Autodesk Inventor part; units mm, degrees
ref_plane "Start Plane" through (0, 0, 20) normal (0, 0, 1) x (1, 0, 0)
ref_plane "End Plane" through (0, 0, 1180) normal (0, 0, 1) x (1, 0, 0)
ref_plane "Work Plane4" through (-800, -15.5, 20) normal (0, 0, -1) x (-1, 0, 0)
ref_plane "Start Plane" through (0, 0, 20) normal (0, 0, 1) x (1, 0, 0)
ref_plane "End Plane" through (0, 0, 1180) normal (0, 0, 1) x (1, 0, 0)
sketch "Sketch" plane through (0, 0, 0) normal (0, 0, 1) x (1, 0, 0)
  line L0 (-20, -15.5) -> (-20, 15.5)
  line L1 (-15.5, 20) -> (15.5, 20)
  line L2 (20, 15.5) -> (20, -15.5)
  line L3 (15.5, -20) -> (-15.5, -20)
  arc A0 (-20, -15.5) -> (-15.5, -20) centre (-15.5, -15.5) ccw
  arc A1 (-15.5, 20) -> (-20, 15.5) centre (-15.5, 15.5) ccw
  arc A2 (20, 15.5) -> (15.5, 20) centre (15.5, 15.5) ccw
  arc A3 (15.5, -20) -> (20, -15.5) centre (15.5, -15.5) ccw
  arc A4 (-15.5, 17) -> (-17, 15.5) centre (-15.5, 15.5) ccw
  line L4 (-15.5, 17) -> (15.5, 17)
  arc A5 (17, 15.5) -> (15.5, 17) centre (15.5, 15.5) ccw
  line L5 (17, 15.5) -> (17, -15.5)
  arc A6 (15.5, -17) -> (17, -15.5) centre (15.5, -15.5) ccw
  line L6 (15.5, -17) -> (-15.5, -17)
  arc A7 (-17, -15.5) -> (-15.5, -17) centre (-15.5, -15.5) ccw
  line L7 (-17, -15.5) -> (-17, 15.5)
  line L8 (0, 29.3048) -> (0, -29.3048) construction
  line L9 (-29.3048, 0) -> (29.3048, 0) construction
  dimension "d7" = 4.5
  dimension "d10" = 40
  dimension "d11" = 40
  dimension "d12" = 3
  dimension "d15" = 20
  dimension "d16" = 20
extrude "Body" add sketch "Sketch" along normal up to surface (1160 mm away) from surface at 20
sketch "Sketch3" plane through (0, 0, 0) normal (0, 0, 1) x (1, 0, 0)
  line L0 (0, 0) -> (10, 0)
ref_plane "Work Plane3" through (0, 0, 0) normal (0, -1, 0) x (1, 0, 0)
ref_plane "Work Plane4" through (-800, -15.5, 20) normal (0, 0, -1) x (-1, 0, 0)
split "Split1" plane through (-800, -15.5, 20) removes the side toward (0, 0, -1)
ref_plane "Work Plane5" through (-500, -984.5, 1180) normal (0, 0, 1) x (1, 0, 0)
split "Split2" plane through (-500, -984.5, 1180) removes the side toward (0, 0, 1)
sketch "Sketch4" plane through (0, 0, 0) normal (0, -1, 0) x (1, 0, 0)
  line L0 (-2, 20) -> (12, 20)
  line L1 (-2, 1180) -> (12, 1180)
  dimension "d18" = 1160
equation "\"d7\" = G_IR"
equation "\"d10\" = G_H"
equation "\"d11\" = G_W"
equation "\"d12\" = G_T"
equation "\"d15\" = 0.5 * d10"
equation "\"d16\" = 0.5 * d11"
equation "\"d3\" = G_L"
equation "\"G_W\" = 40"
equation "\"G_H\" = 40"
equation "\"G_T\" = 3"
equation "\"G_IR\" = 4.5"
equation "\"G_L\" = d18"
properties part number "ISO 12633-2 - 40x40x3 - 1160" material "Steel, Mild"
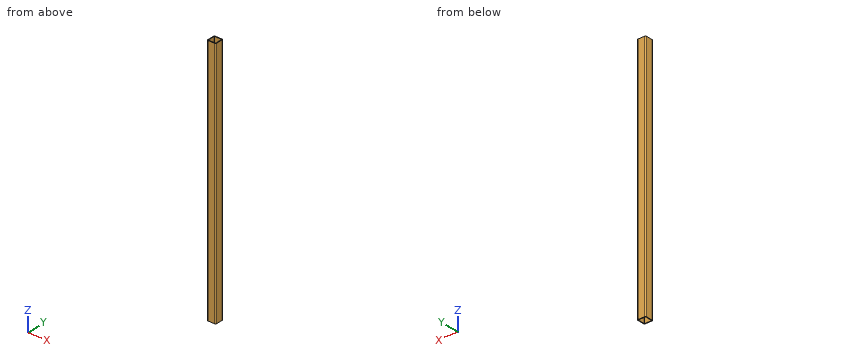
Work out the finished part from the listing and answer in its coordinate system (mm). Coordinates: 2 decimals unless noted, no trailing zeros. Loops run counter-clockwise (first coordinate to the right, second up) from the corner with the lowest first, then second, coordinate; pieces in that order, holes last. Notation, with made-up numbers: M -22.5,83 L 25.5,83 A20 ccw 25.5,99 Z; hole C 36.5,-34.75 d11. An arc over 180 degrees is marked long. Answer in a Markdown table with one row per item. Add a question column.
1. A flat-ended cylindrical pin translates along its axis: P1, Ø1, axis at x = 2, y = 15.5, coming from the -Z side. Find the tip coordinate at first contact, or state that the pin passes through.
2. Find section A-A, the plane x = 1.5. Write down the section's boundary in (y, z), then the cut area to 3 significant figures.
3. Find section C-C, the plane z = 1041.5. Write down the section's boundary in (x, y).
4. Consider L1, parallel to X at y = -0.5, z = 991; L2, parallel to Y at x = -16, z = 267.5. Determine where each line is inside the solid, lowest interval first.
Reported:
| question | item | result |
|---|---|---|
| 1 | P1 | passes through |
| 2 | outline | M -20,20 L -17,20 L -17,1180 L -20,1180 Z; M 17,20 L 20,20 L 20,1180 L 17,1180 Z |
| 2 | area | 6,960 mm^2 |
| 3 | outline | M -20,-15.5 A4.5 ccw -15.5,-20 L 15.5,-20 A4.5 ccw 20,-15.5 L 20,15.5 A4.5 ccw 15.5,20 L -15.5,20 A4.5 ccw -20,15.5 Z; hole M -17,-15.5 A1.5 ccw -15.5,-17 L 15.5,-17 A1.5 ccw 17,-15.5 L 17,15.5 A1.5 ccw 15.5,17 L -15.5,17 A1.5 ccw -17,15.5 Z |
| 4 | L1 | x = -20 to -17, 17 to 20 |
| 4 | L2 | y = -19.97 to -16.91, 16.91 to 19.97 |
